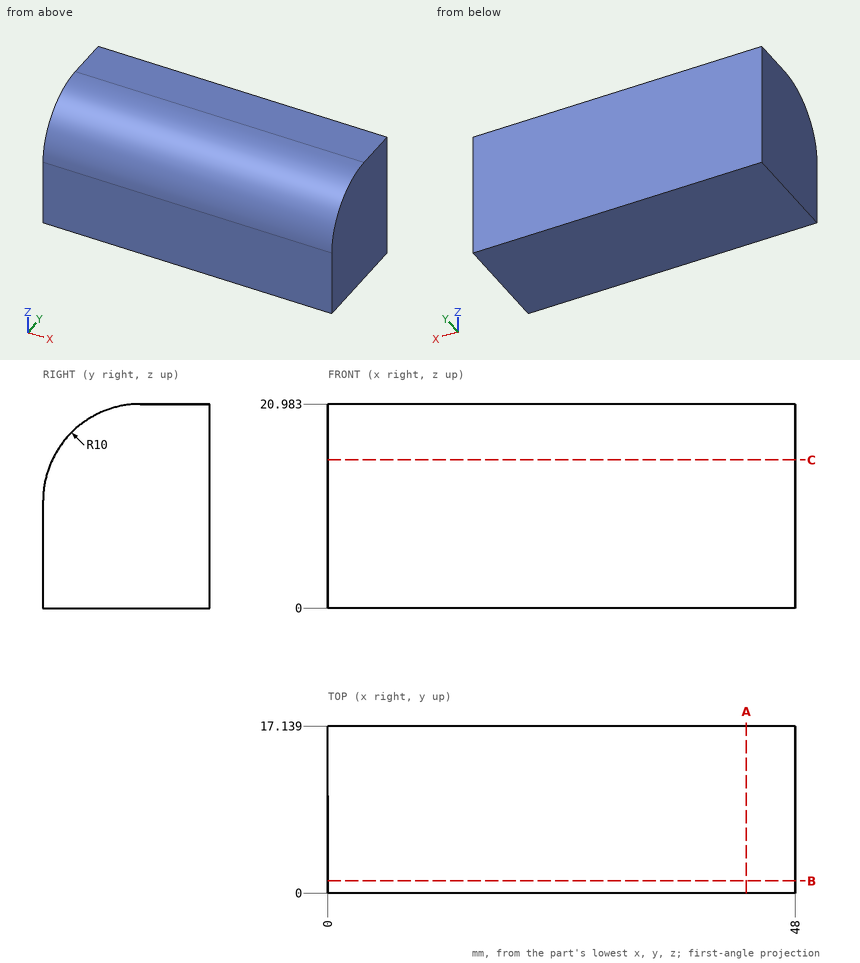
Study the drawing (mm; zero at the part's minimum x, y, z) and answer. Coordinates: 2 decimals unless noted, no trailing zeros. Write each loop counter-clockwise with the first axis right and the second up, starting at its lowest first coordinate (ties: lowest second). Pieces come first, ordered by that corner, then holes. Notation, with made-up numbers: (15.5, 60.5) - (60.5, 60.5) arc R24 cw to (60.5, 94.5) - close; hole circle Ø6 at (82, 43). An arc over 180 degrees is marked (long way). One line per item, written item: value.
1) Find section A-A (x = 43). Give the vertices of the cut face in (y, z).
Geometry check:
outline: (0, 0) - (17.14, 0) - (17.14, 20.98) - (10, 20.98) arc R10 ccw to (0, 10.98) - close
2) Find section C-C (z = 15.25). Give the vertices of the cut face in (x, y).
Geometry check:
outline: (0, 0.96) - (48, 0.96) - (48, 17.14) - (0, 17.14) - close
3) Each of these flat-tipped pins is pushed along its axis until it touches: pin 1 Ø3 at (x, y) = (5.5, 14.5) entering from -Z; pin 2 Ø2 at (x, y) = (17, 4) entering from +Z. Where does it stop, or does it pass through?
Geometry check:
pin 1: stops at z = 0
pin 2: stops at z = 19.64
4) Find section B-B (y = 1.25). Give the vertices of the cut face in (x, z), and give its area (3 significant figures).
Geometry check:
outline: (0, 0) - (48, 0) - (48, 15.82) - (0, 15.82) - close
area: 760 mm2
5) Consider line 1 along Z through (x, y) = (40, 9.75); line 2 along Z through (x, y) = (43.5, 7.75); line 3 along Y through (x, z) = (20, 17.25). Determine where each line is inside the solid, lowest interval first. Write a range as from..to.
Geometry check:
line 1: z = 0..20.98
line 2: z = 0..20.73
line 3: y = 2.21..17.14
